Could you check a few things on this drawing? It's one solid part, dimensions in mm from its lowest x, y, z. Give positions to 0.01 mm unless a question says otherwise; leave off trailing zeros. Loops run counter-clockwise (first coordinate to the right, second up) from the corner with the lowest first, then second, coordinate; pieces in that order, holes last.
1. Imagine slicing it at A-A (z = 3.5). List the corners of the cut face in (x, y) for me.
2. For P1, Ø1.1, axis at y = 2.5, z = 4.5, coming from the -X side, with a flat end and sliding along its axis, tell me the tip position at first contact or that it passes through.
3. Thinking about a two-plate mould opening in X: for the marked faces 1, 2 and 3, which applies, +X half, -X half, draft (parallel to the pull), parting line (faces both ways), or undercut?
4. Imagine slicing it at D-D (x = 23.5). List the corners of the cut face in (y, z) for me, plus the area to 3 significant figures.
5. I need wall thicknesses on line 1 along X through (y, z) = (1.6, 3.5); line 2 along Z through (x, y) = (35, 1.5); line 3 along X through (y, z) = (0.8, 3) (1 decimal). Which ranges of each line are inside material? Lowest first, please.
6. Imagine slicing it at C-C (z = 1.75). List the corners of the cut face in (x, y) for me.
7. Imagine slicing it at B-B (y = 2.5). List the corners of the cut face in (x, z) for me, plus the area to 3 significant figures.
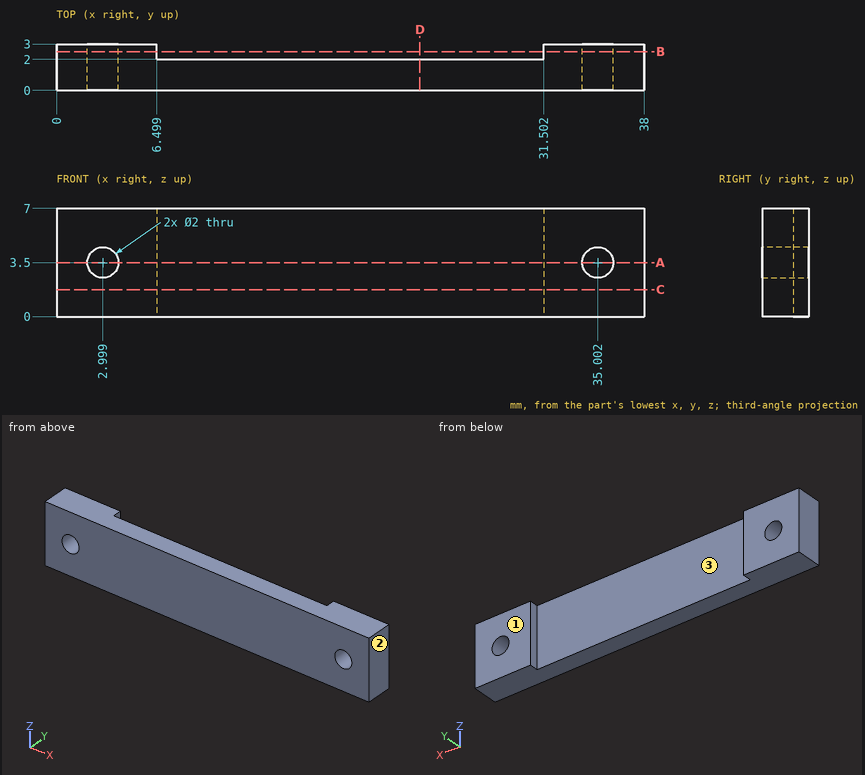
Derived:
1. outline: (0, 0) - (2, 0) - (2, 3) - (0, 3) - close; (4, 0) - (34, 0) - (34, 3) - (31.5, 3) - (31.5, 2) - (6.5, 2) - (6.5, 3) - (4, 3) - close; (36, 0) - (38, 0) - (38, 3) - (36, 3) - close
2. P1: stops at x = 0
3. face 1: draft
3. face 2: +X half
3. face 3: undercut
4. outline: (0, 0) - (2, 0) - (2, 7) - (0, 7) - close
4. area: 14.0 mm2
5. line 1: x = 0 to 2, 4 to 34, 36 to 38
5. line 2: z = 0 to 2.5, 4.5 to 7
5. line 3: x = 0 to 2.1, 3.9 to 34.1, 35.9 to 38
6. outline: (0, 0) - (38, 0) - (38, 3) - (31.5, 3) - (31.5, 2) - (6.5, 2) - (6.5, 3) - (0, 3) - close
7. outline: (0, 0) - (6.5, 0) - (6.5, 7) - (0, 7) - close; (31.5, 0) - (38, 0) - (38, 7) - (31.5, 7) - close; hole circle Ø2 at (3, 3.5); hole circle Ø2 at (35, 3.5)
7. area: 84.7 mm2
